from build123d import *

# Parameters (mm, degrees)
F1_DEPTH     = 25
F2_T1_DEPTH  = 4.6076951546
F2_T3_DEPTH  = 4.6076951546
F2_T5_DEPTH  = 4.6076951546
F2_T8_ANGLE  = 120
F2_T10_ANGLE = 120
F2_T12_ANGLE = 120
F2_T14_ANGLE = 120
F2_T16_ANGLE = 120
F2_T18_ANGLE = 120


# Not quite as in the source:
# - a fillet or chamfer that OpenCascade refuses, or shapes differently, is made with other operations: its cross-section is extruded or revolved along the edge and cut away or added


with BuildPart() as f1:
    # F0 (on Top) → F1 (new body)
    with BuildSketch(Plane.XY):
        with BuildLine():
            Line((-2.3038475773, -4.3301270189), (2.3038475773, -4.3301270189))
            ThreePointArc((2.3038475773, -4.3301270189), (4.9019237886, -2.8301270189), (4.9019237886, 0.1698729811))
            Line((4.9019237886, 0.1698729811), (2.5980762114, 4.1602540378))
            ThreePointArc((2.5980762114, 4.1602540378), (0, 5.6602540378), (-2.5980762114, 4.1602540378))
            Line((-2.5980762114, 4.1602540378), (-4.9019237886, 0.1698729811))
            ThreePointArc((-4.9019237886, 0.1698729811), (-4.9019237886, -2.8301270189), (-2.3038475773, -4.3301270189))
        make_face()
        with BuildLine():
            ThreePointArc((3.25, -1.45), (2.9571067812, -2.1571067812), (2.25, -2.45))
            Line((2.25, -2.45), (-2.25, -2.45))
            ThreePointArc((-2.25, -2.45), (-2.9571067812, -2.1571067812), (-3.25, -1.45))
            Line((-3.25, -1.45), (-3.25, 1.45))
            ThreePointArc((-3.25, 1.45), (-2.9571067812, 2.1571067812), (-2.25, 2.45))
            Line((-2.25, 2.45), (2.25, 2.45))
            ThreePointArc((2.25, 2.45), (2.9571067812, 2.1571067812), (3.25, 1.45))
            Line((3.25, 1.45), (3.25, -1.45))
        make_face(mode=Mode.SUBTRACT)
    extrude(amount=F1_DEPTH)

    # F2: fillet of radius 2 on 12 edges, made by hand

    # F2_s2 → F2_t1 (cut)
    with BuildSketch(Plane(origin=(1.1519237886, -1.9951905284, 0), x_dir=(0, 0, 1), z_dir=(-0.5, 0.8660254038, 0))):
        with BuildLine():
            ThreePointArc((23, 4.3301270189), (24.4142135624, 3.7443405813), (25, 2.3301270189))
            Line((25, 2.3301270189), (25, 4.3301270189))
            Line((25, 4.3301270189), (23, 4.3301270189))
        make_face()
        with BuildLine():
            ThreePointArc((2, 4.3301270189), (0.5857864376, 3.7443405813), (0, 2.3301270189))
            Line((0, 2.3301270189), (0, 4.3301270189))
            Line((0, 4.3301270189), (2, 4.3301270189))
        make_face()
    extrude(amount=F2_T1_DEPTH, mode=Mode.SUBTRACT)

    # F2_s4 → F2_t3 (cut)
    with BuildSketch(Plane(origin=(1.1519237886, 1.9951905284, 0), x_dir=(0, 0, 1), z_dir=(-0.5, -0.8660254038, 0))):
        with BuildLine():
            ThreePointArc((23, 4.3301270189), (24.4142135624, 3.7443405813), (25, 2.3301270189))
            Line((25, 2.3301270189), (25, 4.3301270189))
            Line((25, 4.3301270189), (23, 4.3301270189))
        make_face()
        with BuildLine():
            ThreePointArc((2, 4.3301270189), (0.5857864376, 3.7443405813), (0, 2.3301270189))
            Line((0, 2.3301270189), (0, 4.3301270189))
            Line((0, 4.3301270189), (2, 4.3301270189))
        make_face()
    extrude(amount=F2_T3_DEPTH, mode=Mode.SUBTRACT)

    # F2_s6 → F2_t5 (cut)
    with BuildSketch(Plane.YZ.offset(-2.3038475773)):
        with BuildLine():
            ThreePointArc((-4.3301270189, 23), (-3.7443405813, 24.4142135624), (-2.3301270189, 25))
            Line((-2.3301270189, 25), (-4.3301270189, 25))
            Line((-4.3301270189, 25), (-4.3301270189, 23))
        make_face()
        with BuildLine():
            ThreePointArc((-4.3301270189, 2), (-3.7443405813, 0.5857864376), (-2.3301270189, 0))
            Line((-2.3301270189, 0), (-4.3301270189, 0))
            Line((-4.3301270189, 0), (-4.3301270189, 2))
        make_face()
    extrude(amount=F2_T5_DEPTH, mode=Mode.SUBTRACT)

    # F2_s7 → F2_t8 (revolve, cut)
    with BuildSketch(Plane(origin=(-1.1519237886, 1.9951905284, 0), x_dir=(0, 0, 1), z_dir=(0.5, -0.8660254038, 0))):
        with BuildLine():
            ThreePointArc((23, -4.3301270189), (24.4142135624, -3.7443405813), (25, -2.3301270189))
            Line((25, -2.3301270189), (25, -4.3301270189))
            Line((25, -4.3301270189), (23, -4.3301270189))
        make_face()
    revolve(axis=Axis((0, 2.6602540378, 25), (0, 0, 1)), revolution_arc=F2_T8_ANGLE, mode=Mode.SUBTRACT)

    # F2_s9 → F2_t10 (revolve, cut)
    with BuildSketch(Plane(origin=(-1.1519237886, -1.9951905284, 0), x_dir=(0, 0, 1), z_dir=(0.5, 0.8660254038, 0))):
        with BuildLine():
            ThreePointArc((23, -4.3301270189), (24.4142135624, -3.7443405813), (25, -2.3301270189))
            Line((25, -2.3301270189), (25, -4.3301270189))
            Line((25, -4.3301270189), (23, -4.3301270189))
        make_face()
    revolve(axis=Axis((-2.3038475773, -1.3301270189, 25), (0, 0, 1)), revolution_arc=F2_T10_ANGLE, mode=Mode.SUBTRACT)

    # F2_s11 → F2_t12 (revolve, cut)
    with BuildSketch(Plane.YZ.offset(2.3038475773)):
        with BuildLine():
            ThreePointArc((-4.3301270189, 23), (-3.7443405813, 24.4142135624), (-2.3301270189, 25))
            Line((-2.3301270189, 25), (-4.3301270189, 25))
            Line((-4.3301270189, 25), (-4.3301270189, 23))
        make_face()
    revolve(axis=Axis((2.3038475773, -1.3301270189, 25), (0, 0, 1)), revolution_arc=F2_T12_ANGLE, mode=Mode.SUBTRACT)

    # F2_s13 → F2_t14 (revolve, cut)
    with BuildSketch(Plane.YZ.offset(2.3038475773)):
        with BuildLine():
            ThreePointArc((-4.3301270189, 2), (-3.7443405813, 0.5857864376), (-2.3301270189, 0))
            Line((-2.3301270189, 0), (-4.3301270189, 0))
            Line((-4.3301270189, 0), (-4.3301270189, 2))
        make_face()
    revolve(axis=Axis((2.3038475773, -1.3301270189, 0), (0, 0, 1)), revolution_arc=F2_T14_ANGLE, mode=Mode.SUBTRACT)

    # F2_s15 → F2_t16 (revolve, cut)
    with BuildSketch(Plane(origin=(-1.1519237886, 1.9951905284, 0), x_dir=(0, 0, 1), z_dir=(0.5, -0.8660254038, 0))):
        with BuildLine():
            ThreePointArc((2, -4.3301270189), (0.5857864376, -3.7443405813), (0, -2.3301270189))
            Line((0, -2.3301270189), (0, -4.3301270189))
            Line((0, -4.3301270189), (2, -4.3301270189))
        make_face()
    revolve(axis=Axis((0, 2.6602540378, 0), (0, 0, 1)), revolution_arc=F2_T16_ANGLE, mode=Mode.SUBTRACT)

    # F2_s17 → F2_t18 (revolve, cut)
    with BuildSketch(Plane(origin=(-1.1519237886, -1.9951905284, 0), x_dir=(0, 0, 1), z_dir=(0.5, 0.8660254038, 0))):
        with BuildLine():
            ThreePointArc((2, -4.3301270189), (0.5857864376, -3.7443405813), (0, -2.3301270189))
            Line((0, -2.3301270189), (0, -4.3301270189))
            Line((0, -4.3301270189), (2, -4.3301270189))
        make_face()
    revolve(axis=Axis((-2.3038475773, -1.3301270189, 0), (0, 0, 1)), revolution_arc=F2_T18_ANGLE, mode=Mode.SUBTRACT)


solid = f1.part
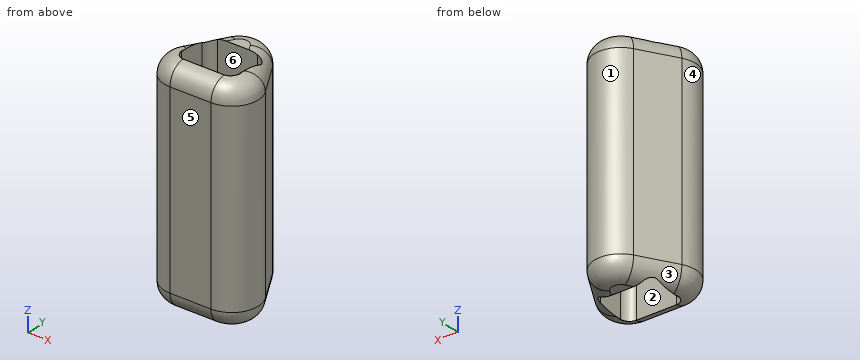
Input: part model. Units: mm. Frame: model coordinates. Face numbers are marked on the shaded views. A direction names the side the tool comes from. Coordinates: 2 decimals unless noted, no trailing zeros. Loops run counter-clockwise (first coordinate to the right, second up) from the corner with the lowest first, then second, coordinate; pieces in that order, holes last. Notation, with made-up numbers: (28.25, -4) - (58.25, -4) arc R19 cw to (58.25, 26) - close; hole circle Ø1 at (65.5, 20.5). An arc over 180 degrees is marked (long way). Answer in a Markdown table with one row per item. Add a question column.
Item 1: Access query for the marked faces 1 and 2. Directions: +Z, -Z, +X, -X, +Y, -Y. A direction counts if a zero-diameter tool reaches every point of the face in a straight line with its end or side. Return the directions, or none.
Item 2: Contact query for flat-ended pins moving along their axis: P1, Ø1.5, axis at x = 0.5, y = -2, coming from the -Z side; P2, Ø1.5, axis at y = 0.5, z = 17, coming from the -X side; P3, Ø1.5, axis at y = 1, z = 6.5, coming from the -X side. Output: stop coordinate, or through.
Item 3: Section query A-A on z = 3.5. Return the cut outline in (x, y), then the cut area to 3 significant figures.
Item 4: Line query: line 1 along X through (y, z) = (-1.25, 13); line 2 along Y through (x, z) = (2, 13); line 3 along X through (y, z) = (0.5, 21.75). Output: solid intervals per line, ascending. Write a range as [from, to].
Item 5: Mould query, pull axis Y, two halves, no side actions, for the marked faces 3, 4, 5 and 6. Classes: released by +Y, released by -Y, zero draft, split by the parting line, or undercut.
Recorded:
| question | item | result |
|---|---|---|
| 1 | face 1 | +Z, -Z, +Y |
| 1 | face 2 | +Z, -Z |
| 2 | P1 | z = 0 |
| 2 | P2 | x = -5.1 |
| 2 | P3 | x = -4.86 |
| 3 | outline | (-4.9, 0.17) arc R3 ccw to (-2.3, -4.33) - (2.3, -4.33) arc R3 ccw to (4.9, 0.17) - (2.6, 4.16) arc R3 ccw to (-2.6, 4.16) - close; hole (-3.25, -1.45) arc R1 ccw to (-2.25, -2.45) - (2.25, -2.45) arc R1 ccw to (3.25, -1.45) - (3.25, 1.45) arc R1 ccw to (2.25, 2.45) - (-2.25, 2.45) arc R1 ccw to (-3.25, 1.45) - close |
| 3 | area | 47.9 mm^2 |
| 4 | line 1 | [-5.3, -3.25], [3.25, 5.3] |
| 4 | line 2 | [-4.33, -2.45], [2.45, 4.9] |
| 4 | line 3 | [-4.71, -3.25], [3.25, 4.71] |
| 5 | face 3 | released by +Y |
| 5 | face 4 | split by the parting line |
| 5 | face 5 | released by -Y |
| 5 | face 6 | undercut |
